Verification items for the finished model (mm, model axes). Give positions to 0.01 mm unless a question says otherwise; leave off trailing zeros. Write each loop counter-clockwise with the first axis right and the second up, starting at its lowest first coordinate (ties: lowest second). Pieces come first, ordered by that corner, then holes.
from build123d import *

# Parameters (mm, degrees)
SKETCH2_R                                       = 4.7625
SKETCH2_W                                       = 6.01
SKETCH2_H                                       = 6.01
SKETCH2_R_2                                     = 5
BOSS_EXTRUDE1_DEPTH                             = 6.35
CSK_FOR_M3_FLAT_HEAD_MACHINE_SCREW1_D           = 3.2
CSK_FOR_M3_FLAT_HEAD_MACHINE_SCREW1_CSINK_D     = 6.3
CSK_FOR_M3_FLAT_HEAD_MACHINE_SCREW1_CSINK_ANGLE = 90
FILLET1_R                                       = 10


with BuildPart() as part:
    # Sketch2 → Boss-Extrude1 (new body)
    with BuildSketch(Plane(origin=(0, 0, 0), x_dir=(1, 0, 0), z_dir=(0, 1, 0))):
        with BuildLine():
            Line((83.085046789, -58.336309448), (12.374368671, 12.374368671))
            Line((12.374368671, 12.374368671), (-22.604233169, 36.514530504))
            ThreePointArc((-22.604233169, 36.514530504), (-35.355339059, 35.355339059), (-36.514530504, 22.604233169))
            Line((-36.514530504, 22.604233169), (-12.374368671, -12.374368671))
            Line((-12.374368671, -12.374368671), (58.336309448, -83.085046789))
            ThreePointArc((58.336309448, -83.085046789), (83.085046789, -83.085046789), (83.085046789, -58.336309448))
        make_face()
        with Locations((70.710678119, -70.710678119)):
            Circle(SKETCH2_R, mode=Mode.SUBTRACT)
        Rectangle(SKETCH2_W, SKETCH2_H, mode=Mode.SUBTRACT)
        with Locations((-28.284271247, 28.284271247)):
            Circle(SKETCH2_R_2, mode=Mode.SUBTRACT)
    extrude(amount=-BOSS_EXTRUDE1_DEPTH)

    # CSK for M3 Flat Head Machine Screw1 (through all)
    with Locations(Plane(origin=(0, 0, -10), x_dir=(0, 0, 1), z_dir=(0, 1, 0))):
        with Locations((0, 0), (10, -10), (10, 10), (20, 0)):
            CounterSinkHole(CSK_FOR_M3_FLAT_HEAD_MACHINE_SCREW1_D / 2, CSK_FOR_M3_FLAT_HEAD_MACHINE_SCREW1_CSINK_D / 2, counter_sink_angle=CSK_FOR_M3_FLAT_HEAD_MACHINE_SCREW1_CSINK_ANGLE)

    # Fillet1
    fillet1_edges = [part.edges().sort_by_distance(p)[0] for p in [
        (12.374368671, -3.175, -12.374368671),
        (-12.374368671, -3.175, 12.374368671),
    ]]
    fillet(fillet1_edges, radius=FILLET1_R)


solid = part.part
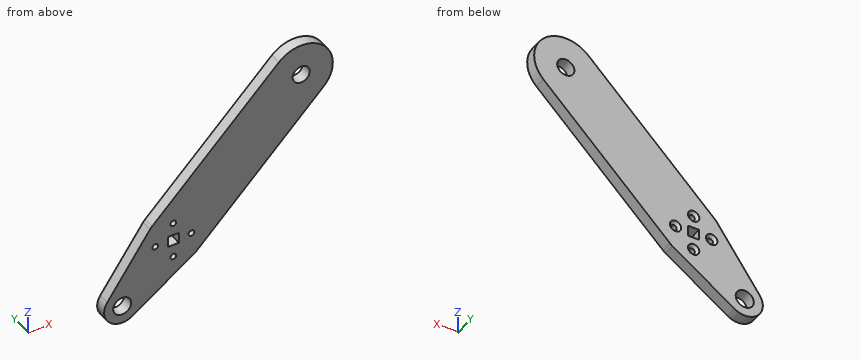
Item 1: Sectioned sample at A-A on z = -10. Record the cut outline in (x, y), then the cut area to 3 significant figures.
Answer key:
outline: (-27.82, -6.35) - (-1.6, -6.35) - (-1.6, -1.55) - (-3.15, 0) - (-27.82, 0) - close; (1.6, -6.35) - (14.75, -6.35) - (14.75, 0) - (3.15, 0) - (1.6, -1.55) - close
area: 248 mm2
Item 2: Sectioned sample at C-C on x = 10. Record the cut outline in (y, z).
Answer key:
outline: (-6.35, -14.01) - (0, -14.01) - (0, -3.15) - (-1.55, -1.6) - (-6.35, -1.6) - close; (-6.35, 1.6) - (-1.55, 1.6) - (0, 3.15) - (0, 34.75) - (-6.35, 34.75) - close
Item 3: Scan lines: line 1 along X through (y, z) = (-2.55, 0) (3 decimals); line 2 along X through (y, z) = (-0.25, 75). Record each from-to range of solid material in increasing order.
Answer key:
line 1: x = -20.914 to -11.6, -8.4 to -3.005, 3.005 to 8.4, 11.6 to 24.749
line 2: x = 50.25 to 68.64, 72.78 to 87.68
Item 4: Sectioned sample at B-B on y = -3.25. Record the cut outline in (x, z) (1 decimal).
Answer key:
outline: (-36.5, -22.6) arc R10 ccw to (-22.6, -36.5) - (11.6, -12.9) arc R10 ccw to (13, -11.7) - (83.1, 58.3) arc R17.5 ccw to (58.3, 83.1) - (-11.7, 13) arc R10 ccw to (-12.9, 11.6) - close; hole circle Ø10 at (-28.3, -28.3); hole circle Ø3.2 at (-10, 0); hole (-3, -3) - (3, -3) - (3, 3) - (-3, 3) - close; hole circle Ø3.2 at (0, -10); hole circle Ø3.2 at (0, 10); hole circle Ø3.2 at (10, 0); hole circle Ø9.5 at (70.7, 70.7)
Item 5: Depth check by flat-ended pin: pin 1 (3 mm diameter, centred on y = -4, z = 12.5, fed in from +X); pin 2 (1.8 mm diameter, centred on x = 0.5, y = -3.5, fed in from -Z); pin 3 (3 mm diameter, centred on x = -10, z = 0, fed in from -Y); pin 4 (1.8 mm diameter, centred on x = 1.5, y = -4.5, fed in from +Z). Enter the tip coordinate at first touch or a pass-through.
Answer key:
pin 1: stops at x = 38.75
pin 2: stops at z = -21.19
pin 3: passes through
pin 4: stops at z = 27.15
Item 6: Sectioned sample at D-D on z = 74. Record the cut outline in (x, y), then the cut area to 3 significant figures.
Answer key:
outline: (49.25, -6.35) - (67.27, -6.35) - (67.27, 0) - (49.25, 0) - close; (74.15, -6.35) - (87.9, -6.35) - (87.9, 0) - (74.15, 0) - close
area: 202 mm2
